For this review, take the finished solid that the model builds, in its own axes (mm). A direction names the side the tool comes from. Give positions to 0.01 mm unless a question says otherwise; leave off trailing zeros. Loops run counter-clockwise (first coordinate to the right, second up) from the corner with the lowest first, then second, coordinate; pieces in that order, holes last. Notation, with made-up numbers: (50.5, 69.25) - (63.5, 69.25) arc R27 cw to (63.5, 105.25) - close; hole circle Ø10 at (12, 3). An arc over 180 degrees is marked (long way). Put each result on its own line as item: value. Start each with the question number.
from build123d import *

# Parameters (mm, degrees)
F0_W     = 914.4
F0_H     = 419.1
F1_DEPTH = 6.35
F2_W     = 88.9
F2_H     = 50.8
F3_DEPTH = 127
F4_W     = 114.3
F4_H     = 114.3
F5_DEPTH = 6.35


with BuildPart() as f1:
    # F0 (on Top) → F1 (new body)
    with BuildSketch(Plane.XY):
        with Locations((8.092676, -162.5851)):
            Rectangle(F0_W, F0_H)
    extrude(amount=F1_DEPTH)

    # F2 (on face) → F3 (join)
    with BuildSketch(Plane(origin=(0, 0, 0), x_dir=(1, 0, 0), z_dir=(0, 0, -1))):
        with Locations((-346.515909, 299.105746)):
            Rectangle(F2_W, F2_H)
        with Locations((-346.515909, 26.064454)):
            Rectangle(F2_W, F2_H)
        with Locations((362.701261, 299.105746)):
            Rectangle(F2_W, F2_H)
        with Locations((362.701261, 26.064454)):
            Rectangle(F2_W, F2_H)
    extrude(amount=F3_DEPTH)

    # F4 (on face) → F5 (cut)
    with BuildSketch(Plane.XY.offset(6.35)):
        with Locations((-36.357324, -162.5851)):
            Rectangle(F4_W, F4_H)
    extrude(amount=-F5_DEPTH, mode=Mode.SUBTRACT)


solid = f1.part
1) Machinability: for faces 5 (the flat face through (407.151, -26, -63)), 6 (the flat face through (-347, -51.464, -63)), 7 (the flat face through (318.251, -26, -63)), 8 (the flat face through (-347, -0.664, -63)), which of the approach directions +Z, -Z, +X, -X, +Y, -Y give a long, thin tool a straight path to every point of the face, cutting with its end or side? Answer none if there is none.
2) Take a section at D-D on x = -316. State the section outline as (y, z) points, and give its area (3 significant figures).
3) Insertion check: P1, Ø10, axis at x = -88, y = -14.5, coming from the -Z side; P2, Ø15, axis at y = -294, z = -46, coming from the +X side; P3, Ø15, axis at y = -291, z = -65.5, coming from the -X side. Each pin has a flat end and moves straight along its axis. Give the tip position at first contact, or say it passes through.
4) Mouldability with a two-part tool opening along Y and no side actions: class faces 1 (the flat face through (-347, -324.506, -63)), 2 (the flat face through (-347, -273.706, -63)), 3 (the flat face through (362, -273.706, -63)), 4 (the flat face through (407.151, -299, -63)) as released by +Y, released by -Y, zero draft, split by the parting line, or undercut.
5) Wall thickness on probe 1 along Y at (x, z) = (-308, -114); probe 2 along Z at (x, y) = (-198, -39); probe 3 along X at (y, z) = (-300, -68): over which ranges is each line inside the solid? List them lowest first.
6) Take a section at A-A on z = -43. State the section outline as (x, y) points.
7) Take a section at B-B on x = -17.5. State the section outline as (y, z) points, and give its area (3 significant figures).
8) Take a section at C-C on y = -173. State the section outline as (x, z) points, and give its area (3 significant figures).
Answers follow:
1. face 5: -Z, +X, +Y, -Y
1. face 6: -Z, +X, -X
1. face 7: -Z, +Y, -Y
1. face 8: -Z, +X, -X, +Y
2. outline: (-372.14, 0) - (-324.51, 0) - (-324.51, -127) - (-273.71, -127) - (-273.71, 0) - (-51.46, 0) - (-51.46, -127) - (-0.66, -127) - (-0.66, 0) - (46.96, 0) - (46.96, 6.35) - (-372.14, 6.35) - close
2. area: 15,600 mm2
3. P1: z = 0
3. P2: x = 407.15
3. P3: x = -390.97
4. face 1: released by -Y
4. face 2: undercut
4. face 3: undercut
4. face 4: zero draft
5. probe 1: -324.51 to -273.71, -51.46 to -0.66
5. probe 2: 0 to 6.35
5. probe 3: -390.97 to -302.07, 318.25 to 407.15
6. outline: (-390.97, -324.51) - (-302.07, -324.51) - (-302.07, -273.71) - (-390.97, -273.71) - close; (-390.97, -51.46) - (-302.07, -51.46) - (-302.07, -0.66) - (-390.97, -0.66) - close; (318.25, -324.51) - (407.15, -324.51) - (407.15, -273.71) - (318.25, -273.71) - close; (318.25, -51.46) - (407.15, -51.46) - (407.15, -0.66) - (318.25, -0.66) - close
7. outline: (-372.14, 0) - (-219.74, 0) - (-219.74, 6.35) - (-372.14, 6.35) - close; (-105.44, 0) - (46.96, 0) - (46.96, 6.35) - (-105.44, 6.35) - close
7. area: 1,940 mm2
8. outline: (-449.11, 0) - (-93.51, 0) - (-93.51, 6.35) - (-449.11, 6.35) - close; (20.79, 0) - (465.29, 0) - (465.29, 6.35) - (20.79, 6.35) - close
8. area: 5,080 mm2
